Work out the finished part from the listing and answer in its coordinate system (mm). A direction names the side the tool comes from. Coordinates: 2 decimals unless noted, no trailing zeros. Order: outer loops, then holes, each group sorted by start corner. A loop starts at its lowest first (then second) coordinate and runs counter-clockwise, first axis right, second up. Notation, with made-up numbers: (-1, 49.25) -> (47, 49.25) arc R30 ccw to (47, 75.25) -> close; hole circle Ø8 at (-37, -33.5). An arc over 180 degrees is marked (long way). Use one line per item in the form item = value.
from build123d import *

# Parameters (mm, degrees)
SKETCH9_R            = 20
BOSS_EXTRUDE8_DEPTH  = 1
SKETCH10_R           = 20
BOSS_EXTRUDE9_DEPTH  = 1
SKETCH11_R           = 18
BOSS_EXTRUDE10_DEPTH = 1
SKETCH13_R           = 17.5
BOSS_EXTRUDE11_DEPTH = 2
FILLET2_R            = 10
SKETCH15_R           = 11.5
BOSS_EXTRUDE14_DEPTH = 1
SKETCH16_R           = 10.5
BOSS_EXTRUDE15_DEPTH = 7
SKETCH17_R           = 1.25
CUT_EXTRUDE1_DEPTH   = 7
SKETCH22_R           = 19.885430157
CUT_EXTRUDE4_DEPTH   = 1
SKETCH23_R           = 18.006686429
CUT_EXTRUDE5_DEPTH   = 1
SKETCH24_R           = 17.498830581
CUT_EXTRUDE6_DEPTH   = 1
SKETCH25_R           = 11.431585712
CUT_EXTRUDE7_DEPTH   = 1
CUT_EXTRUDE8_DEPTH   = 3
SKETCH32_R           = 10.520449086
CUT_EXTRUDE10_DEPTH  = 1


with BuildPart() as part:
    # Sketch9 → Boss-Extrude8 (new body)
    with BuildSketch(Plane.XY):
        with BuildLine():
            Line((16.902313625, 8.740359897), (1.902313625, 8.740359897))
            ThreePointArc((1.902313625, 8.740359897), (16.044449248, 2.882495521), (21.902313625, -11.259640103))
            Line((21.902313625, -11.259640103), (21.902313625, 3.740359897))
            Line((21.902313625, 3.740359897), (16.902313625, 8.740359897))
        make_face()
        with BuildLine():
            ThreePointArc((21.902313625, -11.259640103), (16.044449248, -25.401775727), (1.902313625, -31.259640103))
            Line((1.902313625, -31.259640103), (16.902313625, -31.259640103))
            Line((16.902313625, -31.259640103), (21.902313625, -26.259640103))
            Line((21.902313625, -26.259640103), (21.902313625, -11.259640103))
        make_face()
        with Locations((1.902313625, -11.259640103)):
            Circle(SKETCH9_R)
        with BuildLine():
            ThreePointArc((1.902313625, -31.259640103), (-12.239821999, -25.401775727), (-18.097686375, -11.259640103))
            Line((-18.097686375, -11.259640103), (-18.097686375, -26.259640103))
            Line((-18.097686375, -26.259640103), (-13.097686375, -31.259640103))
            Line((-13.097686375, -31.259640103), (1.902313625, -31.259640103))
        make_face()
        with BuildLine():
            Line((-13.097686375, 8.740359897), (-18.097686375, 3.740359897))
            Line((-18.097686375, 3.740359897), (-18.097686375, -11.259640103))
            ThreePointArc((-18.097686375, -11.259640103), (-12.239821999, 2.882495521), (1.902313625, 8.740359897))
            Line((1.902313625, 8.740359897), (-13.097686375, 8.740359897))
        make_face()
    extrude(amount=BOSS_EXTRUDE8_DEPTH)

    # Sketch10 → Boss-Extrude9 (add)
    with BuildSketch(Plane(origin=(0, 0, 0), x_dir=(-1, 0, 0), z_dir=(0, 0, -1))):
        with Locations((-1.902313625, -11.259640103)):
            Circle(SKETCH10_R)
    extrude(amount=BOSS_EXTRUDE9_DEPTH)

    # Sketch11 → Boss-Extrude10 (add)
    with BuildSketch(Plane(origin=(0, 0, -1), x_dir=(-1, 0, 0), z_dir=(0, 0, -1))):
        with Locations((-1.902313625, -11.259640103)):
            Circle(SKETCH11_R)
    extrude(amount=BOSS_EXTRUDE10_DEPTH)

    # Sketch13 → Boss-Extrude11 (add)
    with BuildSketch(Plane(origin=(0, 0, -2), x_dir=(-1, 0, 0), z_dir=(0, 0, -1))):
        with Locations((-1.902313625, -11.259640103)):
            Circle(SKETCH13_R)
    extrude(amount=BOSS_EXTRUDE11_DEPTH)

    # Fillet2
    # the kernel refuses this fillet: 10 mm, written as the material it takes off along each edge
    with BuildSketch(Plane(origin=(1.902313625, -11.259640103, -4), x_dir=(-1, 0, 0), z_dir=(0, -1, 0))) as fillet2_piece_1:
        with BuildLine():
            CenterArc((11.5, -10), FILLET2_R, 53.130102354, 36.869897646)
            Line((11.5, 0), (11.5, 0.2))
            Line((11.5, 0.2), (17.5, 0.2))
            Line((17.5, 0.2), (17.7, 0))
            ThreePointArc((17.7, 0), (17.7, -1), (17.62, -1.84))
            Line((17.62, -1.84), (17.5, -2))
        make_face()
    revolve(axis=Axis((1.902313625, -11.259640103, -4), (0, 0, -1)), mode=Mode.SUBTRACT)

    # Sketch15 → Boss-Extrude14 (add)
    with BuildSketch(Plane(origin=(0, 0, -4), x_dir=(-1, 0, 0), z_dir=(0, 0, -1))):
        with Locations((-1.902313625, -11.259640103)):
            Circle(SKETCH15_R)
    extrude(amount=BOSS_EXTRUDE14_DEPTH)

    # Sketch16 → Boss-Extrude15 (add)
    with BuildSketch(Plane(origin=(0, 0, -5), x_dir=(-1, 0, 0), z_dir=(0, 0, -1))):
        with Locations((-1.902313625, -11.259640103)):
            Circle(SKETCH16_R)
    extrude(amount=BOSS_EXTRUDE15_DEPTH)

    # Sketch17 → Cut-Extrude1 (cut)
    with BuildSketch(Plane(origin=(0, 0, 0), x_dir=(-1, 0, 0), z_dir=(0, 0, -1))):
        with Locations((-17.988100062, -27.34542654)):
            Circle(SKETCH17_R)
        with Locations((-17.763809056, 5.050437341)):
            Circle(SKETCH17_R)
        with Locations((14.183472813, 4.826146335)):
            Circle(SKETCH17_R)
        with Locations((14.192917147, -27.335982207)):
            Circle(SKETCH17_R)
    extrude(amount=-CUT_EXTRUDE1_DEPTH, mode=Mode.SUBTRACT)

    # Sketch22 → Cut-Extrude4 (cut)
    with BuildSketch(Plane.XY.offset(1)):
        with Locations((1.787515975, -11.354824182)):
            Circle(SKETCH22_R)
    extrude(amount=-CUT_EXTRUDE4_DEPTH, mode=Mode.SUBTRACT)

    # Sketch23 → Cut-Extrude5 (cut)
    with BuildSketch(Plane.XY):
        with Locations((1.870004869, -11.231695531)):
            Circle(SKETCH23_R)
    extrude(amount=-CUT_EXTRUDE5_DEPTH, mode=Mode.SUBTRACT)

    # Sketch24 → Cut-Extrude6 (cut)
    with BuildSketch(Plane.XY.offset(-1)):
        with Locations((2.003621261, -11.194132882)):
            Circle(SKETCH24_R)
    extrude(amount=-CUT_EXTRUDE6_DEPTH, mode=Mode.SUBTRACT)

    # Sketch25 → Cut-Extrude7 (cut)
    with BuildSketch(Plane.XY.offset(-2)):
        with Locations((1.760347749, -11.251117152)):
            Circle(SKETCH25_R)
    extrude(amount=-CUT_EXTRUDE7_DEPTH, mode=Mode.SUBTRACT)

    # Sketch31 → Cut-Extrude8 (cut)
    with BuildSketch(Plane.XY.offset(-2)):
        with BuildLine():
            ThreePointArc((-8.801904408, -1.059495183), (-13.015152024, -11.339263863), (-8.954990434, -21.680452743))
            ThreePointArc((-8.954990434, -21.680452743), (-7.360251179, -21.727858352), (-7.312845569, -20.133119097))
            ThreePointArc((-7.312845569, -20.133119097), (-10.758916086, -11.356013725), (-7.182913489, -2.631038874))
            ThreePointArc((-7.182913489, -2.631038874), (-7.206637103, -1.035771569), (-8.801904408, -1.059495183))
        make_face()
        with BuildLine():
            ThreePointArc((12.532818581, -22.441763104), (17.191560153, -11.705450505), (12.894068467, -0.819503305))
            ThreePointArc((12.894068467, -0.819503305), (10.807683124, -0.784645409), (10.772825228, -2.871030753))
            ThreePointArc((10.772825228, -2.871030753), (14.240965704, -11.656153997), (10.481291133, -20.320519865))
            ThreePointArc((10.481291133, -20.320519865), (10.446433238, -22.406905208), (12.532818581, -22.441763104))
        make_face()
    extrude(amount=-CUT_EXTRUDE8_DEPTH, mode=Mode.SUBTRACT)

    # Sketch32 → Cut-Extrude10 (cut)
    with BuildSketch(Plane.XY.offset(-3)):
        with Locations((1.909022751, -11.226091394)):
            Circle(SKETCH32_R)
    extrude(amount=-CUT_EXTRUDE10_DEPTH, mode=Mode.SUBTRACT)


solid = part.part
(1) Section D-D on z = -7.25 is taken. Write down the section's boundary in (x, y), plus the area to 3 significant figures.
Data:
outline = circle Ø21 at (1.9, -11.26)
area = 346 mm²
(2) The mould has two halves that part along Y. Classify faces 6 (the cylindrical face through (0.5, -0.8, -3.5)), 7 (the flat face through (2, -11, -12)), 8 (the cylindrical face through (4.18, -21.51, -8.45)): released by +Y, released by -Y, zero draft, split by the parting line, or undercut.
Data:
face_6 = undercut
face_7 = zero draft
face_8 = split by the parting line
(3) Section A-A on z = -2.5 is taken. Count the separate pieces of the cut face and the enclosed holes in it, plus the area to 3 significant figures.
Data:
separate_pieces = 1
enclosed_holes = 3
area = 350 mm²
(4) Straight lines are drawn through the part: line 1 along X through (y, z) = (-9, -2.25); line 2 along Z through (x, y) = (-11, 2); line 3 along Y through (x, z) = (-5.5, -2.75). For each, find the intervals that lie inside material, in ascending order.
Data:
line_1 = -15.1 to -12.81, -10.52 to -9.45, 12.97 to 14, 17 to 18.9
line_2 = -1 to 0
line_3 = -25.83 to -20.08, -2.42 to 3.31
(5) Each of these flat-tipped pins is pushed along its axis until it touches: P1, Ø18.5, axis at x = -3.5, y = -11.5, coming from the +Z side; P2, Ø22, axis at x = 16, y = -24, coming from the -Z side; P3, Ø10, axis at x = 17, y = 2.5, coming from the -Z side; P4, Ø3, axis at x = -14.18, y = 4.83, coming from the -Z side. Where does it stop, or does it pass through?
Data:
P1 = -2
P2 = -12
P3 = -3.2
P4 = 0
(6) Which of the six approach directions +Z, -Z, +X, -X, +Y, -Y give full straight-line access (tool end or side, diameter ignored) to faces 1 (the flat face through (17, -26, 0)), 2 (the flat face through (-3, -21, -5)), 3 (the flat face through (-15.5, -13.8, -1)), 4 (the flat face through (19.437, 6.205, 0.493)), 5 (the cylindrical face through (17.188, -11.874, -2.644))?
Data:
face_1 = -Z, +X, -Y
face_2 = -Z
face_3 = +Z
face_4 = +Z, -Z, +X, +Y
face_5 = +Z, -Z
